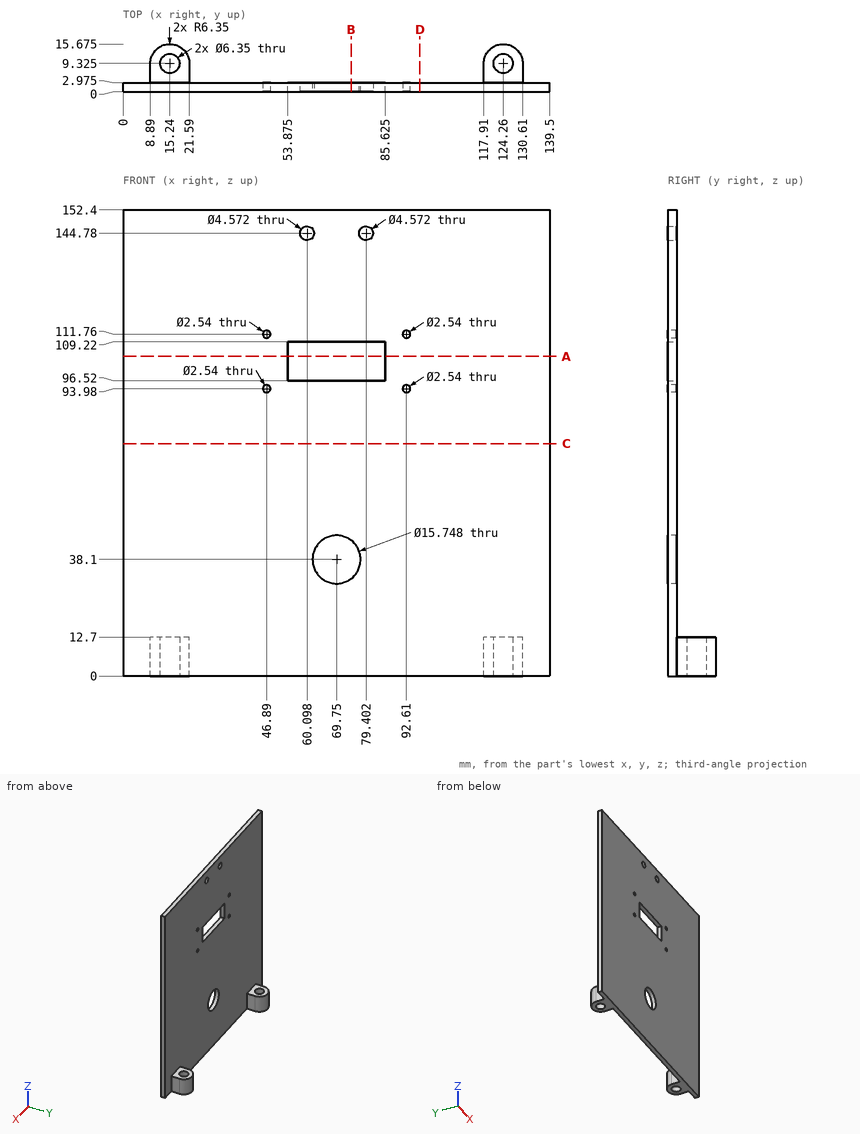
Drawing for the job (mm, zero at the part's lowest x, y, z). Give positions to 0.01 mm unless a question says otherwise; leave off trailing zeros. Write each loop counter-clockwise with the first axis right and the second up, starting at its lowest first coordinate (ties: lowest second). Pieces come first, ordered by that corner, then holes. Notation, with made-up numbers: (76, 19) - (124, 19) arc R17 cw to (124, 39) - close; hole circle Ø9 at (21, 27). An arc over 180 degrees is marked (long way). Answer as CSV lines item,"result".
Q1. Flat gauge pins, fed straight in: pin 1 Ø10 at (x, z) = (39.5, 48) entering from +Y (3 decimals); pin 2 Ø3.5 at (x, z) = (46.89, 111.76) entering from -Y; pin 3 Ø1.9 at (y, z) = (6, 5) entering from -X. Where does each tip first touch, or does it go through?
Result set:
pin 1,"y = 2.975"
pin 2,"y = 0"
pin 3,"x = 8.89"
Q2. Band-saw the part on C-C (z = 76). Give the cut face in (x, y) (3 decimals).
Result set:
outline,"(0, 0) - (139.5, 0) - (139.5, 2.975) - (0, 2.975) - close"
Q3. Band-saw the part on A-A (z = 104.5). Give the cut face in (x, y) (3 decimals), and give its area (3 significant figures).
Result set:
outline,"(0, 0) - (53.875, 0) - (53.875, 2.975) - (0, 2.975) - close; (85.625, 0) - (139.5, 0) - (139.5, 2.975) - (85.625, 2.975) - close"
area,"321 mm²"
Q4. Band-saw the part on D-D (x = 97). Give the cut face in (y, z) (3 decimals).
Result set:
outline,"(0, 0) - (2.975, 0) - (2.975, 152.4) - (0, 152.4) - close"
Q5. Drill centre lines: line 1 (Z direction, x = 46.89, y = 2.15); line 2 (X direction, y = 2.3, z = 144.78); line 3 (X direction, y = 1.05, z = 93.98). Where is each one in solid material? Low to high. Write a range as from..to.
Result set:
line 1,"0..92.71, 95.25..110.49, 113.03..152.4"
line 2,"0..57.81, 62.38..77.12, 81.69..139.5"
line 3,"0..45.62, 48.16..91.34, 93.88..139.5"
Q6. Band-saw the part on B-B (x = 74.5). Give the cut face in (y, z) (3 decimals), and give its area (3 significant figures).
Result set:
outline,"(0, 0) - (2.975, 0) - (2.975, 31.82) - (0, 31.82) - close; (0, 44.38) - (2.975, 44.38) - (2.975, 96.52) - (0, 96.52) - close; (0, 109.22) - (2.975, 109.22) - (2.975, 152.4) - (0, 152.4) - close"
area,"378 mm²"
